Read the model definition and answer for the solid it produces. Units are mm, in the model's axes. A direction names the side the tool comes from. Round coordinates to 2 decimals unless told otherwise and drop trailing zeros. Order: outer loops, then holes, each group sorted by start corner. A loop starts at its lowest first (then second) coordinate and runs counter-clockwise, first axis right, second up. Notation, with made-up numbers: (10, 29.5) -> (48, 29.5) arc R22 ccw to (48, 36.5) -> close; hole circle Ø9 at (-22, 24). An arc over 180 degrees is marked (long way). Answer as a JSON object with one key per item and string values. Group by question number.
Item 1: Section A-A, the plane z = 21.65 is taken. Write down the section's boundary in (x, y) (3 decimals), plus the area to 4 significant figures.
Item 2: Section B-B, the plane x = -22 is taken. Write down the section's boundary in (y, z).
Item 3: Consider probe 1 along Z at (x, y) = (6.5, -9.5); probe 2 along Z at (x, y) = (17.5, -7.75); probe 3 along Y at (x, z) = (-37.5, -6.5). Determine where each line is inside the solid, lowest interval first. Write a range as from..to.
Item 4: Given P1, Ø6, axis at x = -29.025, z = 21.65, coming from the -Y side; P2, Ø4, axis at y = -9, z = 0.5, coming from the -X side; P3, Ø3.5, axis at x = -39, y = -2.5, coming from the +Z side; P4, Ø3.5, axis at x = -39.48, z = 0, coming from the -Y side, each flat-ended and moving along its own axis, determine where each tip first touches the part or whether it passes through.
Item 5: The mould has two halves that part along X. Classify faces 4 (the flat face through (-4, -9, 5.91)), 5 (the flat face through (-44.3, -2, 0)), 6 (the flat face through (-11, 0, 15)): pulls with the +X half, pulls with the -X half, needs draft (parallel to the pull), parting line crosses it, or undercut.
Item 6: For faces 1 (the flat face through (33, -5, -13.65)), 2 (the flat face through (0, -4, -14.15)), 3 (the flat face through (-29, -4.5, 19)), determine the directions among +Z, -Z, +X, -X, +Y, -Y from which every point of the face is accessible in a straight line to the end or side of a thin tool.
Item 7: Section C-C, the plane y = -7.25 is taken. Write down the section's boundary in (x, z).
Item 8: Section D-D, the plane z = 8.91 is taken. Write down the section's boundary in (x, y), plus the area to 4 significant figures.
from build123d import *

# Parameters (mm, degrees)
F0_R     = 1.95
F1_DEPTH = 10
F2_DEPTH = 8.5
F3_R     = 1.95
F4_DEPTH = 5.5
F6_DEPTH = 25


with BuildPart() as f1:
    # F0 (on Front) → F1 (new body)
    with BuildSketch(Plane.XZ):
        with BuildLine():
            Line((-34.3, 23.65), (-34.3, 16.65))
            Line((-34.3, 16.65), (-23.75, 16.65))
            Line((-23.75, 16.65), (-23.75, 23.65))
            ThreePointArc((-23.75, 23.65), (-24.62868, 25.77132), (-26.75, 26.65))
            Line((-26.75, 26.65), (-31.3, 26.65))
            ThreePointArc((-31.3, 26.65), (-33.42132, 25.77132), (-34.3, 23.65))
        make_face()
        with Locations((-29.025, 21.65)):
            Circle(F0_R, mode=Mode.SUBTRACT)
        with BuildLine():
            Line((23.75, 16.65), (34.3, 16.65))
            Line((34.3, 16.65), (34.3, 23.65))
            ThreePointArc((34.3, 23.65), (33.42132, 25.77132), (31.3, 26.65))
            Line((31.3, 26.65), (26.75, 26.65))
            ThreePointArc((26.75, 26.65), (24.62868, 25.77132), (23.75, 23.65))
            Line((23.75, 23.65), (23.75, 16.65))
        make_face()
        with Locations((29.025, 21.65)):
            Circle(F0_R, mode=Mode.SUBTRACT)
        with BuildLine():
            Line((34.3, 16.65), (34.3, 6.1))
            Line((34.3, 6.1), (41.3, 6.1))
            ThreePointArc((41.3, 6.1), (43.42132, 6.97868), (44.3, 9.1))
            Line((44.3, 9.1), (44.3, 13.65))
            ThreePointArc((44.3, 13.65), (43.42132, 15.77132), (41.3, 16.65))
            Line((41.3, 16.65), (34.3, 16.65))
        make_face()
        with Locations((39.3, 11.375)):
            Circle(F0_R, mode=Mode.SUBTRACT)
        with BuildLine():
            Line((-31.8, 11.91), (-31.8, 14.15))
            Line((-31.8, 14.15), (31.8, 14.15))
            Line((31.8, 14.15), (31.8, 0))
            Line((31.8, 0), (34.3, 0))
            Line((34.3, 0), (34.3, 6.1))
            Line((34.3, 6.1), (34.3, 16.65))
            Line((34.3, 16.65), (23.75, 16.65))
            Line((23.75, 16.65), (-23.75, 16.65))
            Line((-23.75, 16.65), (-34.3, 16.65))
            Line((-34.3, 16.65), (-34.3, -16.65))
            Line((-34.3, -16.65), (31.3, -16.65))
            ThreePointArc((31.3, -16.65), (33.42132, -15.77132), (34.3, -13.65))
            Line((34.3, -13.65), (31.8, -13.65))
            Line((31.8, -13.65), (31.8, -14.15))
            Line((31.8, -14.15), (-31.8, -14.15))
            Line((-31.8, -14.15), (-31.8, 5.91))
            Line((-31.8, 5.91), (-31.8, 11.91))
        make_face()
        with BuildLine():
            Line((-41.3, -16.65), (-34.3, -16.65))
            Line((-34.3, -16.65), (-34.3, 16.65))
            Line((-34.3, 16.65), (-41.3, 16.65))
            ThreePointArc((-41.3, 16.65), (-43.42132, 15.77132), (-44.3, 13.65))
            Line((-44.3, 13.65), (-44.3, -13.65))
            ThreePointArc((-44.3, -13.65), (-43.42132, -15.77132), (-41.3, -16.65))
        make_face()
        with Locations((-39.483927, 0)):
            Circle(F0_R, mode=Mode.SUBTRACT)
        with BuildLine():
            Line((31.8, 14.15), (-31.8, 14.15))
            Line((-31.8, 14.15), (-31.8, 11.91))
            Line((-31.8, 11.91), (23.8, 11.91))
            ThreePointArc((23.8, 11.91), (26.8, 8.91), (23.8, 5.91))
            Line((23.8, 5.91), (-31.8, 5.91))
            Line((-31.8, 5.91), (-31.8, -14.15))
            Line((-31.8, -14.15), (31.8, -14.15))
            Line((31.8, -14.15), (31.8, -13.65))
            Line((31.8, -13.65), (31.8, 0))
            Line((31.8, 0), (31.8, 14.15))
        make_face()
    extrude(amount=F1_DEPTH)

    # F0 (on Front) → F2 (cut)
    with BuildSketch(Plane.XZ):
        with BuildLine():
            Line((31.8, 14.15), (-31.8, 14.15))
            Line((-31.8, 14.15), (-31.8, 11.91))
            Line((-31.8, 11.91), (23.8, 11.91))
            ThreePointArc((23.8, 11.91), (26.8, 8.91), (23.8, 5.91))
            Line((23.8, 5.91), (-31.8, 5.91))
            Line((-31.8, 5.91), (-31.8, -14.15))
            Line((-31.8, -14.15), (31.8, -14.15))
            Line((31.8, -14.15), (31.8, -13.65))
            Line((31.8, -13.65), (31.8, 0))
            Line((31.8, 0), (31.8, 14.15))
        make_face()
    extrude(amount=F2_DEPTH, mode=Mode.SUBTRACT)

    # F3 (on face) → F4 (cut)
    with BuildSketch(Plane.XZ.offset(10)):
        with BuildLine():
            ThreePointArc((-31.3, 26.65), (-33.42132, 25.77132), (-34.3, 23.65))
            Line((-34.3, 23.65), (-34.3, 16.65))
            Line((-34.3, 16.65), (-23.75, 16.65))
            Line((-23.75, 16.65), (-23.75, 23.65))
            ThreePointArc((-23.75, 23.65), (-24.62868, 25.77132), (-26.75, 26.65))
            Line((-26.75, 26.65), (-31.3, 26.65))
        make_face()
        with Locations((-29.025, 21.65)):
            Circle(F3_R, mode=Mode.SUBTRACT)
        with BuildLine():
            Line((-34.3, -16.65), (-34.3, 16.65))
            Line((-34.3, 16.65), (-41.3, 16.65))
            ThreePointArc((-41.3, 16.65), (-43.42132, 15.77132), (-44.3, 13.65))
            Line((-44.3, 13.65), (-44.3, -13.65))
            ThreePointArc((-44.3, -13.65), (-43.42132, -15.77132), (-41.3, -16.65))
            Line((-41.3, -16.65), (-34.3, -16.65))
        make_face()
        with Locations((-39.483927, 0)):
            Circle(F3_R, mode=Mode.SUBTRACT)
        with BuildLine():
            Line((23.75, 23.65), (23.75, 16.65))
            Line((23.75, 16.65), (34.3, 16.65))
            Line((34.3, 16.65), (34.3, 23.65))
            ThreePointArc((34.3, 23.65), (33.42132, 25.77132), (31.3, 26.65))
            Line((31.3, 26.65), (26.75, 26.65))
            ThreePointArc((26.75, 26.65), (24.62868, 25.77132), (23.75, 23.65))
        make_face()
        with Locations((29.025, 21.65)):
            Circle(F3_R, mode=Mode.SUBTRACT)
        with BuildLine():
            Line((41.3, 16.65), (34.3, 16.65))
            Line((34.3, 16.65), (34.3, 6.1))
            Line((34.3, 6.1), (41.3, 6.1))
            ThreePointArc((41.3, 6.1), (43.42132, 6.97868), (44.3, 9.1))
            Line((44.3, 9.1), (44.3, 13.65))
            ThreePointArc((44.3, 13.65), (43.42132, 15.77132), (41.3, 16.65))
        make_face()
        with Locations((39.3, 11.375)):
            Circle(F3_R, mode=Mode.SUBTRACT)
    extrude(amount=-F4_DEPTH, mode=Mode.SUBTRACT)

    # F5 (on face) → F6 (cut)
    with BuildSketch(Plane.XZ):
        Polygon((52.0982, 24.629619), (34.3, 23.65), (34.3, 16.65), (34.3, 0), (53.583535, -2.356674), align=None)
    extrude(amount=F6_DEPTH, mode=Mode.SUBTRACT)


solid = f1.part
Values found:
{
 "1": {"outline": "(-34.3, -4.5) -> (-30.975, -4.5) -> (-30.975, 0) -> (-34.3, 0) -> close; (-27.075, -4.5) -> (-23.75, -4.5) -> (-23.75, 0) -> (-27.075, 0) -> close; (23.75, -4.5) -> (27.075, -4.5) -> (27.075, 0) -> (23.75, 0) -> close; (30.975, -4.5) -> (34.3, -4.5) -> (34.3, 0) -> (30.975, 0) -> close", "area": "59.85 mm2"},
 "2": {"outline": "(-10, -16.65) -> (0, -16.65) -> (0, -14.15) -> (-8.5, -14.15) -> (-8.5, 5.91) -> (-10, 5.91) -> close; (-10, 11.91) -> (-8.5, 11.91) -> (-8.5, 14.15) -> (0, 14.15) -> (0, 16.65) -> (-10, 16.65) -> close"},
 "3": {"probe 1": "-16.65..5.91, 11.91..16.65", "probe 2": "-16.65..-14.15, 14.15..16.65", "probe 3": "-4.5..0"},
 "4": {"P1": "y = -4.5", "P2": "x = -34.3", "P3": "z = 16.65", "P4": "through"},
 "5": {"face 4": "undercut", "face 5": "pulls with the -X half", "face 6": "needs draft"},
 "6": {"face 1": "+X, +Y, -Y", "face 2": "+Y", "face 3": "+Z, +X, -X, -Y"},
 "7": {"outline": "(-34.3, -16.65) -> (31.3, -16.65) arc R3 ccw to (34.3, -13.65) -> (31.8, -13.65) -> (31.8, -14.15) -> (-31.8, -14.15) -> (-31.8, 14.15) -> (31.8, 14.15) -> (31.8, 0) -> (34.3, 0) -> (34.3, 16.65) -> (-34.3, 16.65) -> close"},
 "8": {"outline": "(-44.3, -4.5) -> (-34.3, -4.5) -> (-34.3, -10) -> (-31.8, -10) -> (-31.8, 0) -> (-44.3, 0) -> close; (26.8, -10) -> (34.3, -10) -> (34.3, 0) -> (31.8, 0) -> (31.8, -8.5) -> (26.8, -8.5) -> close", "area": "102.5 mm2"}
}
